Input: part model. Units: mm. Frame: model coordinates. A direction names the side the tool comes from. Coordinates: 2 decimals unless noted, no trailing zeros. Loops run counter-clockwise (first coordinate to the right, second up) from the corner with the lowest first, then second, coordinate; pieces in that order, holes last. Notation, with made-up numbers: (40, 34.25) -> (84, 34.25) arc R12 ccw to (84, 46.25) -> close; hole circle Ø8 at (20, 53.5). An arc over 180 degrees is marked (long way). Answer as a JSON object with one key per item and string values.
Autodesk Inventor part; units mm, degrees
ref_plane "YZ Plane" through (0, 0, 0) normal (1, 0, 0) x (0, 1, 0)
ref_plane "XZ Plane" through (0, 0, 0) normal (0, 1, 0) x (-1, 0, 0)
ref_plane "XY Plane" through (0, 0, 0) normal (0, 0, 1) x (1, 0, 0)
sketch "Sketch2" plane through (0, 0, 0) normal (0, 1, 0) x (-1, 0, 0)
  line L0 (45, 50) -> (-45, 50)
  line L1 (-45, 50) -> (-45, -50)
  line L2 (-45, -50) -> (45, -50)
  line L3 (45, -50) -> (45, 50)
  line L4 (45, 50) -> (-45, -50) construction
  line L5 (-45, 50) -> (45, -50) construction
  point P0 (0, 0)
  dimension "d0" = 90
  dimension "d1" = 100
extrude "Extrusion1" add sketch "Sketch2" along normal blind 50
sketch "Sketch4" plane through (0, 50, 0) normal (0, 1, 0) x (1, 0, 0)
  point P0 (0, 0)
  point P1 (40.9905, 45.9844)
hole "Hole1" at (40.9905, 50, -45.9844) direction (0, -1, 0) diameter 8 end through all
sketch "Sketch5" plane through (0, 0, 0) normal (0, -1, 0) x (1, 0, 0)
  point P0 (0, 0)
  point P1 (-40.9769, 45.9697)
hole "Hole2" at (-40.9769, 0, 45.9697) direction (0, 1, 0) diameter 8 end through all
sketch "Sketch6" plane through (0, 0, 0) normal (0, -1, 0) x (1, 0, 0)
  point P0 (0, 0)
  point P1 (-40.9656, -45.9539)
hole "Hole3" at (-40.9656, 0, -45.9539) direction (0, 1, 0) diameter 8 end through all
sketch "Sketch7" plane through (0, 50, 0) normal (0, 1, 0) x (1, 0, 0)
  point P0 (0, 0)
  point P1 (40.9483, -45.9561)
hole "Hole4" at (40.9483, 50, 45.9561) direction (0, -1, 0) diameter 8 end through all
thread "Thread1"
thread "Thread2"
thread "Thread3"
thread "Thread4"
fillet "Fillet1" radius 4 1 edges at (45, 25, -50)
fillet "Fillet2" radius 4 1 edges at (-45, 25, -50)
fillet "Fillet3" radius 4 1 edges at (-45, 25, 50)
fillet "Fillet4" radius 4 1 edges at (45, 25, 50)
sketch "Sketch9" plane through (0, 50, 0) normal (0, 1, 0) x (1, 0, 0)
  circle A0 centre (0, 0) radius 30
  dimension "d44" = 60
extrude "Extrusion2" add sketch "Sketch9" along normal blind 50
sketch "Sketch10" plane through (0, 100, 0) normal (0, 1, 0) x (1, 0, 0)
  circle A0 centre (0, 0) radius 25
  dimension "d47" = 50
extrude "Extrusion3" cut sketch "Sketch10" against normal blind 30
thread "Thread5"
fillet "Fillet5" radius 2.5 1 edges at (-30, 100, 0)
properties part number "Práctica 1 - Melany Escobar"
1. Mould query, pull axis Z, two halves, no side actions, for faces 1 (the face through (45, 25, 1)), 2 (the face through (-29.97, 73.42, 1.32)), 3 (the face through (23.846, 85.21, -7.509)). Classes: pulls with the +Z half, pulls with the -Z half, needs draft (parallel to the pull), parting line crosses it, or undercut.
Reply:
{"face 1": "needs draft", "face 2": "parting line crosses it", "face 3": "undercut"}
2. Section query D-D (z = 0). Return loops of the section in (x, y).
Reply:
{"outline": "(-45, 0) -> (45, 0) -> (45, 50) -> (30, 50) -> (30, 97.5) arc R2.5 ccw to (27.5, 100) -> (25, 100) -> (25, 70) -> (-25, 70) -> (-25, 100) -> (-27.5, 100) arc R2.5 ccw to (-30, 97.5) -> (-30, 50) -> (-45, 50) -> close"}
3. Section query A-A (x = 0). Return loops of the section in (y, z).
Reply:
{"outline": "(0, -50) -> (50, -50) -> (50, -30) -> (97.5, -30) arc R2.5 ccw to (100, -27.5) -> (100, -25) -> (70, -25) -> (70, 25) -> (100, 25) -> (100, 27.5) arc R2.5 ccw to (97.5, 30) -> (50, 30) -> (50, 50) -> (0, 50) -> close"}
4. Access query for faces 4 (the face through (-45, 25, -1)), 5 (the face through (0, 70, 0)). Directions: +Z, -Z, +X, -X, +Y, -Y. A direction counts if a zero-diameter tool reaches every point of the face in a straight line with its end or side. Return the directions, or none.
Reply:
{"face 4": "+Z, -Z, -X, +Y, -Y", "face 5": "+Y"}
5. Section query B-B (z = 43.5). Return loops of the section in (x, y), plus the area to 3 significant figures.
Reply:
{"outline": "(-45, 0) -> (-44.12, 0) -> (-44.12, 50) -> (-45, 50) -> close; (-37.83, 0) -> (37.79, 0) -> (37.79, 50) -> (-37.83, 50) -> close; (44.11, 0) -> (45, 0) -> (45, 50) -> (44.11, 50) -> close", "area": "3,870 mm2"}
6. Line query: line 1 along Z through (x, y) = (0, 81); line 2 along Y through (x, z) = (29, 27); line 3 along X through (y, z) = (21, 44.5). Output: solid intervals per line, ascending.
Reply:
{"line 1": "z = -30 to -25, 25 to 30", "line 2": "y = 0 to 50", "line 3": "x = -45 to -44.7, -37.26 to 37.22, 44.67 to 45"}
7. Pin query (flat end, axial travel): P1, Ø12, axis at x = 21.5, y = 88.5, coming from the +Z side; P2, Ø25, axis at x = -7.5, z = -2.5, coming from the +Y side; P3, Ø3, axis at x = 33.5, z = -16, coming from the +Y side; P4, Ø10, axis at x = -13.5, z = -5, coming from the -Y side. Return the tip coordinate at first contact, or that it passes through.
Reply:
{"P1": "stops at z = 25.69", "P2": "stops at y = 70", "P3": "stops at y = 50", "P4": "stops at y = 0"}
8. Section query C-C (y = 43). Return loops of the section in (x, z).
Reply:
{"outline": "(-45, -46) arc R4 ccw to (-41, -50) -> (41, -50) arc R4 ccw to (45, -46) -> (45, 46) arc R4 ccw to (41, 50) -> (-41, 50) arc R4 ccw to (-45, 46) -> close; hole circle Ø8 at (-40.98, 45.97); hole circle Ø8 at (-40.97, -45.95); hole circle Ø8 at (40.95, 45.96); hole circle Ø8 at (40.99, -45.98)"}
